Design review of the part built by this model. Coordinates are the model's own, in mm. Face numbers are marked on the shaded views. A direction names the side the tool comes from. Give positions to 0.01 mm unless a question says otherwise; leave off trailing zeros. Write each loop counter-clockwise with the first axis right and the second up, starting at its lowest first coordinate (ties: lowest second). Pieces come first, ordered by that corner, then holes. Notation, with made-up numbers: M 26.25,56 L 85.25,56 A15 ccw 85.25,78 Z; hole C 49,-40 d10. An arc over 180 degrees is marked long. One line per item, written item: value. Start each with the question number.
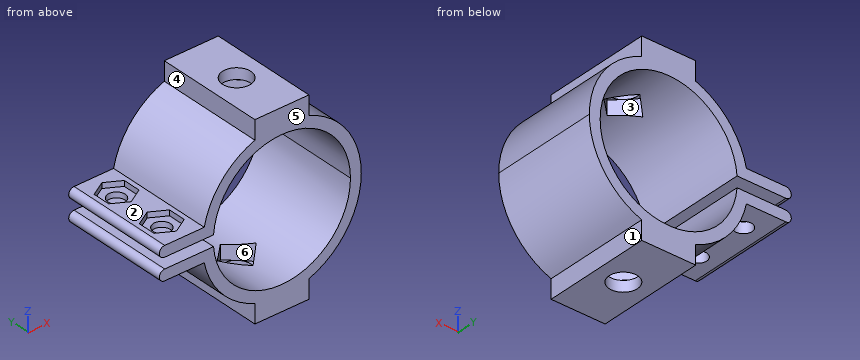
```python
from build123d import *

# Parameters (mm, degrees)
BOSS_EXTRUDE1_DEPTH      = 10
CUT_EXTRUDE10_REACH      = 46.578
CUT_EXTRUDE10_END_RADIUS = 12.7
CUT_EXTRUDE10_START      = -2
SKETCH8_R                = 2.625
CUT_EXTRUDE11_DEPTH      = 2
CUT_EXTRUDE12_DEPTH      = 1
CUT_EXTRUDE13_REACH      = 33.436
SKETCH10_R               = 1.6


# Read off the part's stored shape, not the designer's step: Mirror2
with BuildPart() as part:
    # Sketch1 → Boss-Extrude1 (new, symmetric)
    with BuildSketch(Plane(origin=(0, 0, 0), x_dir=(1, 0, 0), z_dir=(0, 1, 0))):
        with BuildLine():
            Line((-12.709296078, -1.000053339), (-21.709296078, -1.000053339))
            ThreePointArc((-21.709296078, -1.000053339), (-22.709296078, -2.000053339), (-21.709296078, -3.000053339))
            Line((-21.709296078, -3.000053339), (-14.399918025, -3.000053339))
            ThreePointArc((-14.399918025, -3.000053339), (14.690703922, -5.3339e-05), (-14.399918025, 2.999946661))
            Line((-14.399918025, 2.999946661), (-21.709296078, 2.999946661))
            ThreePointArc((-21.709296078, 2.999946661), (-22.709296078, 1.999946661), (-21.709296078, 0.999946661))
            Line((-21.709296078, 0.999946661), (-12.709296078, 0.999946661))
            Line((-12.709296078, 0.999946661), (-12.669864786, 0.999946661))
            ThreePointArc((-12.669864786, 0.999946661), (12.690703922, -5.3339e-05), (-12.669864786, -1.000053339))
            Line((-12.669864786, -1.000053339), (-12.709296078, -1.000053339))
        make_face()
        with BuildLine():
            ThreePointArc((4.990703922, -13.823584002), (-0.009296078, -14.700053339), (-5.009296078, -13.823584002))
            Line((-5.009296078, -13.823584002), (-5.009296078, -14.750053339))
            Line((-5.009296078, -14.750053339), (-5.009296078, -17.300053339))
            Line((-5.009296078, -17.300053339), (4.990703922, -17.300053339))
            Line((4.990703922, -17.300053339), (4.990703922, -14.750053339))
            Line((4.990703922, -14.750053339), (4.990703922, -13.823584002))
        make_face()
        with BuildLine():
            Line((-5.009296078, 14.749946661), (-5.009296078, 13.823477324))
            ThreePointArc((-5.009296078, 13.823477324), (-0.009296078, 14.699946661), (4.990703922, 13.823477324))
            Line((4.990703922, 13.823477324), (4.990703922, 14.749946661))
            Line((4.990703922, 14.749946661), (4.990703922, 17.299946661))
            Line((4.990703922, 17.299946661), (-5.009296078, 17.299946661))
            Line((-5.009296078, 17.299946661), (-5.009296078, 14.749946661))
        make_face()
    extrude(amount=BOSS_EXTRUDE1_DEPTH, both=True)

    # Cut-Extrude10: up to this cylinder (the profile starts outside it)
    cut_extrude10_end = Plane(origin=(-0.009296078, 0, 5.3339e-05), z_dir=(0, -1, 0)) * Cylinder(CUT_EXTRUDE10_END_RADIUS, 119.556, mode=Mode.PRIVATE)
    # Sketch7 → Cut-Extrude10 (cut, up to the surface)
    with BuildSketch(Plane.XY.offset(17.300053339).offset(CUT_EXTRUDE10_START), mode=Mode.PRIVATE) as cut_extrude10_sk1:
        Polygon((0, 3.606244584), (-3.606244584, 0), (0, -3.606244584), (3.606244584, 0), align=None)
    cut_extrude10_tool1 = extrude(cut_extrude10_sk1.sketch, amount=-CUT_EXTRUDE10_REACH, mode=Mode.PRIVATE) - cut_extrude10_end
    add(cut_extrude10_tool1.solids().sort_by_distance((0, 0, 15.300053))[0], mode=Mode.SUBTRACT)

    # Sketch8 → Cut-Extrude11 (cut)
    with BuildSketch(Plane.XY.offset(17.300053339)):
        Circle(SKETCH8_R)
    extrude(amount=-CUT_EXTRUDE11_DEPTH, mode=Mode.SUBTRACT)

    # Mirror2
    split(bisect_by=Plane.XY, keep=Keep.TOP)

    # Mirror2 2: part across plane


with BuildPart() as part_1:
    add(part.part)
    add(part.part.mirror(Plane.XY))

    # Sketch9 → Cut-Extrude12 (cut)
    with BuildSketch(Plane.XY.offset(3.000053339)):
        Polygon((-18.054607052, 8.233161507), (-20.854607052, 6.616580754), (-20.854607052, 3.383419246), (-18.054607052, 1.766838493), (-15.254607052, 3.383419246), (-15.254607052, 6.616580754), align=None)
        Polygon((-18.054607052, -1.766838493), (-20.854607052, -3.383419246), (-20.854607052, -6.616580754), (-18.054607052, -8.233161507), (-15.254607052, -6.616580754), (-15.254607052, -3.383419246), align=None)
    extrude(amount=-CUT_EXTRUDE12_DEPTH, mode=Mode.SUBTRACT)

    # Cut-Extrude13: up to this face of the body (flat: up to its plane)
    cut_extrude13_end = Plane(part_1.part.faces().sort_by_distance((-18.054607052, 0, -3.000053339))[0])
    # Sketch10 → Cut-Extrude13 (cut, up to the picked face)
    with BuildSketch(Plane.XY.offset(2.000053339), mode=Mode.PRIVATE) as cut_extrude13_sk1:
        with Locations((-18.054607052, 5)):
            Circle(SKETCH10_R)
    cut_extrude13_tool1 = split(extrude(cut_extrude13_sk1.sketch, amount=-CUT_EXTRUDE13_REACH, mode=Mode.PRIVATE), bisect_by=cut_extrude13_end, keep=Keep.BOTH, mode=Mode.PRIVATE)
    # Sketch10 → Cut-Extrude13 (cut, up to the picked face)
    with BuildSketch(Plane.XY.offset(2.000053339), mode=Mode.PRIVATE) as cut_extrude13_sk2:
        with Locations((-18.054607052, -5)):
            Circle(SKETCH10_R)
    cut_extrude13_tool2 = split(extrude(cut_extrude13_sk2.sketch, amount=-CUT_EXTRUDE13_REACH, mode=Mode.PRIVATE), bisect_by=cut_extrude13_end, keep=Keep.BOTH, mode=Mode.PRIVATE)
    add(cut_extrude13_tool1.solids().sort_by(Axis((-18.054607, 5, 2.000053), (0, 0, -1)))[0], mode=Mode.SUBTRACT)
    add(cut_extrude13_tool2.solids().sort_by(Axis((-18.054607, -5, 2.000053), (0, 0, -1)))[0], mode=Mode.SUBTRACT)


solid = part_1.part
```
Q1. Take a section at A-A, the plane z = 2.5. Give the boundary of the cut face in (x, y), then the cut area to 3 significant figures.
Q2. The part is to be moulded in two halves that separate along Y. For the marked faces 4, 5 and 6, say which applies: pulls with the +Y half, pulls with the -Y half, needs draft (parallel to the pull), parting line crosses it, or undercut.
Q3. Machinability: for the marked faces 1, 2 and 3, which of the approach directions +Z, -Z, +X, -X, +Y, -Y give a long, thin tool a straight path to every point of the face, cutting with its end or side? Answer none if there is none.
Q4. Take a section at C-C, the plane x = -8. Give the boundary of the cut face in (y, z).
Q5. Take a section at B-B, the plane y = 5. State how many separate pieces and enclosed holes the cut face has, then the cut area to 3 significant figures.
Q6. Take a section at D-D, the plane z = -6. Give the boundary of the cut face in (x, y).
Q7. For P1, Ø4, axis at y = 4, z = -14.5, coming from the -X side (3 decimals); P2, Ø1, axis at y = 5, z = 6, coming from the +X side; P3, Ø12, axis at x = -18.5, y = -2.5, coming from the -Z side, all flat-tipped, find the tip position at first contact; note any pin that passes through.
Q8. Wall thickness on line 1 (X direction, y = 0, z = 15.8) (3 decimals); line 2 (Y direction, x = 0, z = 16) (3 decimals); line 3 (X direction, y = -2.75, z = -8): over which ranges is each line inside the solid? List them lowest first. Write a range as from..to.
Results list:
1. outline: M -22.58,-10 L -12.46,-10 L -12.46,10 L -22.58,10 Z; M 12.44,-10 L 14.48,-10 L 14.48,10 L 12.44,10 Z; hole M -20.85,-6.62 L -18.05,-8.23 L -15.25,-6.62 L -15.25,-3.38 L -18.05,-1.77 L -20.85,-3.38 Z; hole M -20.85,3.38 L -18.05,1.77 L -15.25,3.38 L -15.25,6.62 L -18.05,8.23 L -20.85,6.62 Z
1. area: 189 mm^2
2. face 4: needs draft
2. face 5: pulls with the -Y half
2. face 6: undercut
3. face 1: -Z, +X, +Y, -Y
3. face 2: +Z, -X, +Y, -Y
3. face 3: none
4. outline: M -10,-12.34 L 10,-12.34 L 10,-9.87 L -10,-9.87 Z; M -10,9.87 L 10,9.87 L 10,12.34 L -10,12.34 Z
5. separate pieces: 3
5. enclosed holes: 0
5. area: 242 mm^2
6. outline: M -13.43,-10 L -11.2,-10 L -11.2,10 L -13.43,10 Z; M 11.18,-10 L 13.41,-10 L 13.41,10 L 11.18,10 Z
7. P1: stops at x = -7.745
7. P2: stops at x = 13.62
7. P3: stops at z = -7.75
8. line 1: x = -5.009..-2.625, 2.625..4.991
8. line 2: y = -10..-2.625, 2.625..10
8. line 3: x = -12.34..-9.87, 9.85..12.32
